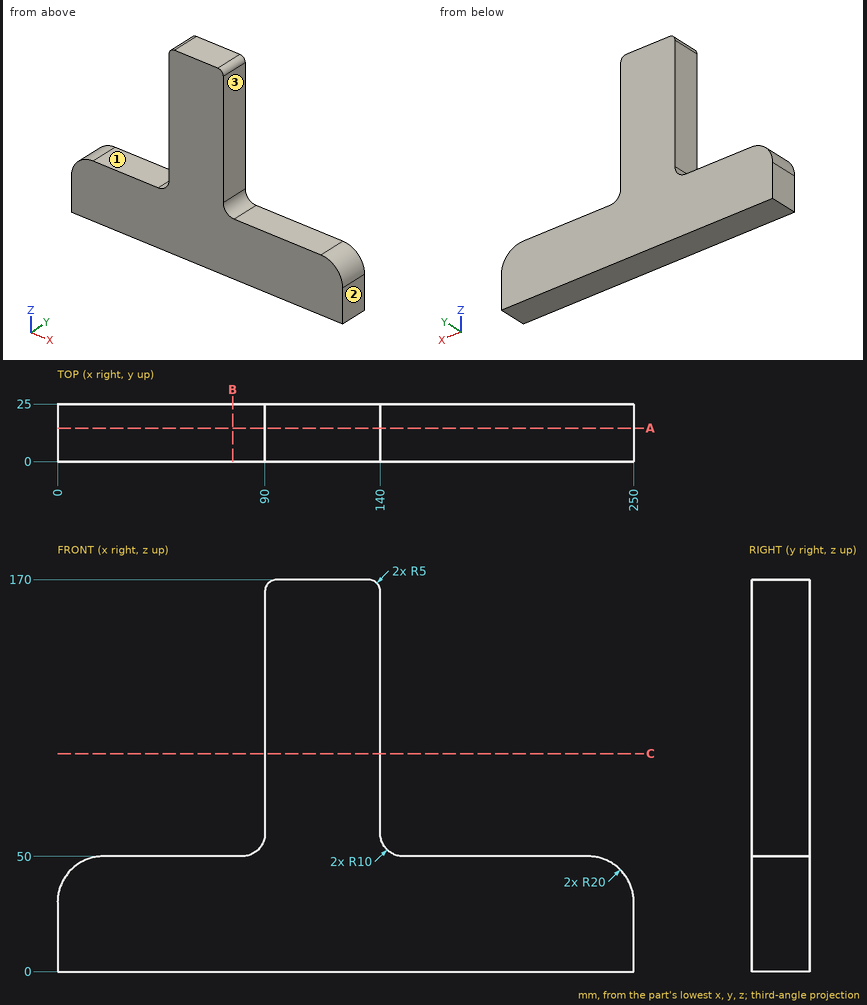
Source: three-view drawing plus pictorial views. Frame: mm from the lowest corner of the part. A direction names the side the tool comes from. Give positions to 0.01 mm unless a question says otherwise; leave off trailing zeros. Write each loop counter-clockwise with the first axis right and the second up, starting at its lowest first coordinate (ties: lowest second). Pieces come first, ordered by that corner, then holes. Notation, with made-up numbers: (-4, -17.75) -> (3, -17.75) arc R26 ccw to (3, 15.25) -> close; hole circle Ø8 at (58, 11). An arc over 180 degrees is marked (long way). Write item = value, one per line.
Q1. Line query: line 1 (Z direction, x = 201, y = 6); line 2 (X direction, y = 11, z = 62); line 3 (Z direction, x = 141, y = 22). Output: solid intervals per line, ascending. Write a range as from..to.
Here are the results:
line_1 = 0..50
line_2 = 90..140
line_3 = 0..55.64
Q2. First-contact query: pin 1 (8 mm diameter, centred on x = 101.5, z = 30, fed in from -Y); pin 2 (7.5 mm diameter, centred on x = 54, y = 11.5, fed in from +Z); pin 3 (3 mm diameter, centred on y = 16, z = 82, fed in from +X). Flat tips, straight axial feed; report the tip coordinate or a pass-through.
Here are the results:
pin_1 = 0
pin_2 = 50
pin_3 = 140
Q3. Cut plane A-A on y = 14.5. Return loops of the section in (x, z), then the cut area to 3 significant figures.
Here are the results:
outline = (0, 0) -> (250, 0) -> (250, 30) arc R20 ccw to (230, 50) -> (150, 50) arc R10 cw to (140, 60) -> (140, 165) arc R5 ccw to (135, 170) -> (95, 170) arc R5 ccw to (90, 165) -> (90, 60) arc R10 cw to (80, 50) -> (20, 50) arc R20 ccw to (0, 30) -> close
area = 18,400 mm²
Q4. Cut plane B-B on x = 76. Return loops of the section in (y, z).
Here are the results:
outline = (0, 0) -> (25, 0) -> (25, 50) -> (0, 50) -> close
Q5. Reachability of the marked faces 1, 2 and 3 from +Z, -Z, +X, -X, +Y, -Y: full face, straight path, thin tool, end or side. Return the list, or none.
Here are the results:
face_1 = +Z, -X, +Y, -Y
face_2 = +Z, -Z, +X, +Y, -Y
face_3 = +Z, +X, +Y, -Y
Q6. Cut plane C-C on z = 94.5. Return loops of the section in (x, y), then the cut area to 3 significant figures.
Here are the results:
outline = (90, 0) -> (140, 0) -> (140, 25) -> (90, 25) -> close
area = 1,250 mm²
